from build123d import *

# Parameters (mm, degrees)
SKETCH1_R           = 4.5
BOSS_EXTRUDE1_DEPTH = 3
FILLET1_R           = 1
BOSS_EXTRUDE2_DEPTH = 1
SKETCH6_R           = 1.75
BOSS_EXTRUDE3_DEPTH = 14


with BuildPart() as part:
    # Sketch1 → Boss-Extrude1 (new body)
    with BuildSketch(Plane(origin=(0, 115.601531763, -5.053e-06), x_dir=(1, 0, 0), z_dir=(0, 1, -4.4e-08))):
        with Locations((40.91030477, -143.155151275)):
            Circle(SKETCH1_R)
    extrude(amount=BOSS_EXTRUDE1_DEPTH)

    # Fillet1
    fillet1_edges = [part.edges().sort_by_distance(p)[0] for p in [
        (36.41030477, 118.601538021, 143.155146091),
    ]]
    fillet(fillet1_edges, radius=FILLET1_R)

    # Sketch2 → Boss-Extrude2 (add)
    with BuildSketch(Plane(origin=(0, 118.601531763, -5.184e-06), x_dir=(1, 0, 0), z_dir=(0, 1, -4.4e-08))):
        Polygon((40.11030477, -142.303288868), (40.11030477, -144.855151275), (41.71030477, -144.855151275), (41.71030477, -142.303288868), (42.41030477, -142.303288868), (40.91030477, -140.803288868), (39.41030477, -142.303288868), align=None)
    extrude(amount=BOSS_EXTRUDE2_DEPTH)

    # Sketch6 → Boss-Extrude3 (add)
    with BuildSketch(Plane(origin=(0, 115.601531763, -5.053e-06), x_dir=(-1, 0, 0), z_dir=(0, -1, 4.4e-08))):
        with Locations((-40.91030477, -143.155151275)):
            Circle(SKETCH6_R)
    extrude(amount=BOSS_EXTRUDE3_DEPTH)


solid = part.part
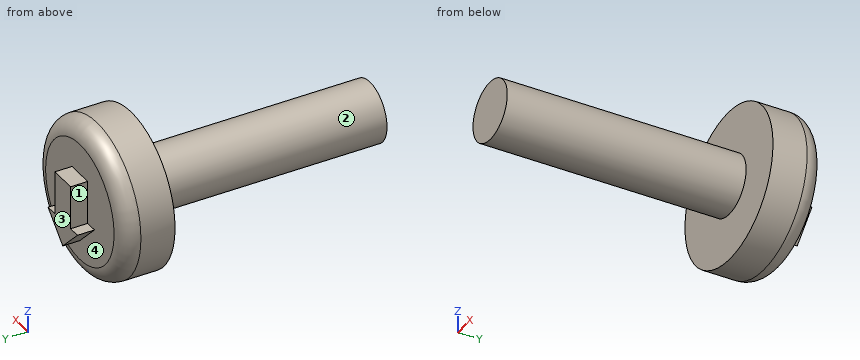
The model under review builds one solid part; all positions refer to its coordinate system, in mm. Face numbers are marked on the shaded views. A direction names the side the tool comes from. Round coordinates to 2 decimals unless told otherwise and drop trailing zeros. Loops run counter-clockwise (first coordinate to the right, second up) from the corner with the lowest first, then second, coordinate; pieces in that order, holes last. Notation, with made-up numbers: (-1.5, 55.25) - (20.5, 55.25) arc R24 ccw to (20.5, 67.25) - close; hole circle Ø7 at (-22, 86). An arc over 180 degrees is marked (long way). Use CSV: the item, a comma, the result in double quotes.
(1) Take a section at B-B, the plane y = 107. Give the boundary of the cut face in (x, z).
Working result:
outline,"circle Ø3.5 at (40.91, 143.16)"
(2) For line 1 (Y direction, x = 44, z = 144.75); line 2 (Z direction, x = 42, y = 103.25); line 3 (Z direction, x = 40, y = 103), list the stretches that pass through material, from the lowest coordinate up.
Working result:
line 1,"y = 115.6 to 118.6"
line 2,"z = 141.79 to 144.52"
line 3,"z = 141.66 to 144.65"
(3) Take a section at A-A, the plane y = 116. Give the boundary of the cut face in (x, z).
Working result:
outline,"circle Ø9 at (40.91, 143.16)"
(4) Machinability: for the marked faces 1, 2, 3 and 4, which of the approach directions +Z, -Z, +X, -X, +Y, -Y give a long, thin tool a straight path to every point of the face, cutting with its end or side? Answer none if there is none.
Working result:
face 1,"+Z, -X, +Y"
face 2,"-Y"
face 3,"+Z, -Z, +X, -X, +Y"
face 4,"+Y"
(5) Clearance check with flat-ended pins moving along their axes: P1, Ø0.5, axis at x = 41, y = 119, coming from the +Z side; P2, Ø3, axis at x = 37.5, z = 139.5, coming from the -Y side; P3, Ø5, axis at y = 117.5, z = 140.5, coming from the +X side. State where each tip first meets the part, or that it passes through.
Working result:
P1,"stops at z = 144.86"
P2,"stops at y = 115.6"
P3,"stops at x = 45.41"
